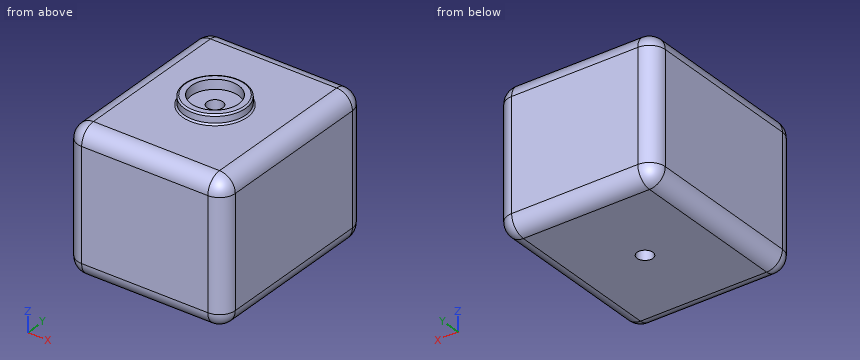
from build123d import *

# Parameters (mm, degrees)
SKETCH1_W           = 10
SKETCH1_H           = 12
BOSS_EXTRUDE1_DEPTH = 9
SKETCH3_R           = 1.95
BOSS_EXTRUDE2_DEPTH = 0.6
SKETCH5_R           = 1.5
CUT_EXTRUDE1_DEPTH  = 0.6
SKETCH7_R           = 0.5
CUT_EXTRUDE2_DEPTH  = 19.027756377
FILLET1_R           = 1
FILLET2_R           = 0.1


with BuildPart() as part:
    # Sketch1 → Boss-Extrude1 (new body)
    with BuildSketch(Plane.XY):
        with Locations((5, 6)):
            Rectangle(SKETCH1_W, SKETCH1_H)
    extrude(amount=-BOSS_EXTRUDE1_DEPTH)

    # Sketch3 → Boss-Extrude2 (add)
    with BuildSketch(Plane.XY):
        with Locations(Location((5, 6, 0), (0, 0, 180))):
            Circle(SKETCH3_R)
    extrude(amount=BOSS_EXTRUDE2_DEPTH)

    # Sketch5 → Cut-Extrude1 (cut)
    with BuildSketch(Plane.XY.offset(0.6)):
        with Locations((5, 6)):
            Circle(SKETCH5_R)
    extrude(amount=-CUT_EXTRUDE1_DEPTH, mode=Mode.SUBTRACT)

    # Sketch7 → Cut-Extrude2 (cut, through all)
    with BuildSketch(Plane.XY):
        with Locations((5, 6)):
            Circle(SKETCH7_R)
    extrude(amount=-CUT_EXTRUDE2_DEPTH, mode=Mode.SUBTRACT)

    # Fillet1
    fillet1_edges = [part.edges().sort_by_distance(p)[0] for p in [
        (10, 6, -9),
        (5, 12, -9),
        (0, 6, -9),
        (5, 12, 0),
        (10, 6, 0),
        (5, 0, 0),
        (0, 6, 0),
        (5, 0, -9),
        (0, 12, -4.5),
        (10, 12, -4.5),
        (10, 0, -4.5),
        (0, 0, -4.5),
    ]]
    fillet(fillet1_edges, radius=FILLET1_R)

    # Fillet2
    fillet2_edges = [part.edges().sort_by_distance(p)[0] for p in [
        (6.95, 6, 0),
        (6.95, 6, 0.6),
    ]]
    fillet(fillet2_edges, radius=FILLET2_R)


solid = part.part
Geometry: final body of the model. Coordinates: model frame, mm. Round coordinates to 2 decimals unless told otherwise and drop trailing zeros. Loops run counter-clockwise (first coordinate to the right, second up) from the corner with the lowest first, then second, coordinate; pieces in that order, holes last. Notation, with made-up numbers: M 84,72.5 L 110,72.5 A14 ccw 110,96.5 Z; hole C -11.5,76 d1. An arc over 180 degrees is marked long. Put each result on its own line as item: value. Start each with the question number.
(1) Section query D-D (x = 7.75). Return loops of the section in (y, z).
(2) Material intervals for line 1 along Y through (x, z) = (5, 0.3); line 2 along Y through (x, z) = (5, -2.75); line 3 along Z through (x, y) = (6.25, 10), sorted ascending. Write a range as [from, to].
(3) Section query A-A (y = 6). Return loops of the section in (x, z).
(4) Contact query for flat-ended pins moving along their axis: pin 1 Ø2.5 at (x, y) = (5, 6) entering from -Z; pin 2 Ø1 at (x, y) = (8, 6.5) entering from +Z. Output: stop coordinate, or through.
(5) Section query B-B (x = 5). Return loops of the section in (y, z), then the cut area to 3 significant figures.
(6) Section query C-C (y = 1.25). Return loops of the section in (x, z).
Findings below:
1. outline: M 0,-8 A1 ccw 1,-9 L 11,-9 A1 ccw 12,-8 L 12,-1 A1 ccw 11,0 L 1,0 A1 ccw 0,-1 Z
2. line 1: y = [4.05, 4.5], [7.5, 7.95]
2. line 2: y = [0, 5.5], [6.5, 12]
2. line 3: z = [-9, 0]
3. outline: M 0,-8 A1 ccw 1,-9 L 4.5,-9 L 4.5,0 L 3.5,0 L 3.5,0.6 L 3.15,0.6 A0.1 ccw 3.05,0.5 L 3.05,0.1 A0.1 cw 2.95,0 L 1,0 A1 ccw 0,-1 Z; M 5.5,-9 L 9,-9 A1 ccw 10,-8 L 10,-1 A1 ccw 9,0 L 7.05,0 A0.1 cw 6.95,0.1 L 6.95,0.5 A0.1 ccw 6.85,0.6 L 6.5,0.6 L 6.5,0 L 5.5,0 Z
4. pin 1: stops at z = -9
4. pin 2: stops at z = 0
5. outline: M 0,-8 A1 ccw 1,-9 L 5.5,-9 L 5.5,0 L 4.5,0 L 4.5,0.6 L 4.15,0.6 A0.1 ccw 4.05,0.5 L 4.05,0.1 A0.1 cw 3.95,0 L 1,0 A1 ccw 0,-1 Z; M 6.5,-9 L 11,-9 A1 ccw 12,-8 L 12,-1 A1 ccw 11,0 L 8.05,0 A0.1 cw 7.95,0.1 L 7.95,0.5 A0.1 ccw 7.85,0.6 L 7.5,0.6 L 7.5,0 L 6.5,0 Z
5. area: 98.7 mm2
6. outline: M 0,-8 A1 ccw 1,-9 L 9,-9 A1 ccw 10,-8 L 10,-1 A1 ccw 9,0 L 1,0 A1 ccw 0,-1 Z
